from build123d import *

# Parameters (mm, degrees)
ESQUISSE1_W                    = 90
ESQUISSE1_H                    = 60
BOSS_EXTRU_1_DEPTH             = 2.7
ESQUISSE2_W                    = 9
ESQUISSE2_H                    = 2.7
BOSS_EXTRU_2_DEPTH             = 2.7
R_P_TITION_LIN_AIRE1_COUNT     = 3
R_P_TITION_LIN_AIRE1_PITCH     = 18
R_P_TITION_LIN_AIRE1_COL_COUNT = 3
R_P_TITION_LIN_AIRE1_COL_PITCH = 18
ESQUISSE3_W                    = 2.7
ESQUISSE3_H                    = 9.8
ENL_V_MAT_EXTRU_1_DEPTH        = 2.7
R_P_TITION_LIN_AIRE2_COUNT     = 5
R_P_TITION_LIN_AIRE2_PITCH     = 20
SYM_TRIE1_COPY_1_SKETCH_W      = 2.7
SYM_TRIE1_COPY_1_SKETCH_H      = 9.8
SYM_TRIE1_COPY_1_DEPTH         = 2.7
SYM_TRIE1_COPY_2_SKETCH_W      = 2.7
SYM_TRIE1_COPY_2_SKETCH_H      = 9.8
SYM_TRIE1_COPY_2_DEPTH         = 2.7
SYM_TRIE1_COPY_3_SKETCH_W      = 2.7
SYM_TRIE1_COPY_3_SKETCH_H      = 9.8
SYM_TRIE1_COPY_3_DEPTH         = 2.7
SYM_TRIE1_COPY_4_SKETCH_W      = 2.7
SYM_TRIE1_COPY_4_SKETCH_H      = 9.8
SYM_TRIE1_COPY_4_DEPTH         = 2.7
ESQUISSE14_W                   = 30
ESQUISSE14_H                   = 20
ENL_V_MAT_EXTRU_4_DEPTH        = 1


with BuildPart() as part:
    # Esquisse1 → Boss.-Extru.1 (new body)
    with BuildSketch(Plane.XY):
        with Locations((0, -30)):
            Rectangle(ESQUISSE1_W, ESQUISSE1_H)
    extrude(amount=BOSS_EXTRU_1_DEPTH)

    # Esquisse2 → Boss.-Extru.2 (add)
    with BuildSketch(Plane.XY):
        with Locations((0, -61.35)):
            Rectangle(ESQUISSE2_W, ESQUISSE2_H)
    boss_extru_2 = extrude(amount=BOSS_EXTRU_2_DEPTH)

    # Répétition linéaire1: Boss.-Extru.2 ×3
    with Locations(*[(i * R_P_TITION_LIN_AIRE1_PITCH, 0, 0) for i in range(1, R_P_TITION_LIN_AIRE1_COUNT)]):
        add(boss_extru_2)

    # Répétition linéaire1 col: Boss.-Extru.2 ×3
    with Locations(*[(-i * R_P_TITION_LIN_AIRE1_COL_PITCH, 0, 0) for i in range(1, R_P_TITION_LIN_AIRE1_COL_COUNT)]):
        add(boss_extru_2)

    # Esquisse3 → Enlèv. mat.-Extru.1 (cut)
    with BuildSketch(Plane.XY):
        with Locations((43.65, -50)):
            Rectangle(ESQUISSE3_W, ESQUISSE3_H)
    enl_v_mat_extru_1 = extrude(amount=ENL_V_MAT_EXTRU_1_DEPTH, mode=Mode.SUBTRACT)

    # Répétition linéaire2: Enlèv. mat.-Extru.1 ×5
    with Locations(*[(0, i * R_P_TITION_LIN_AIRE2_PITCH, 0) for i in range(1, R_P_TITION_LIN_AIRE2_COUNT)]):
        add(enl_v_mat_extru_1, mode=Mode.SUBTRACT)

    # Symétrie1: Enlèv. mat.-Extru.1 across plane
    add(enl_v_mat_extru_1.mirror(Plane(origin=(0, 0, 0), x_dir=(0, 0, 1), z_dir=(1, 0, 0))), mode=Mode.SUBTRACT)

    # Symétrie1 copy 1 sketch → Symétrie1 copy 1 (cut)
    with BuildSketch(Plane(origin=(0, 20, 0), x_dir=(-1, 0, 0), z_dir=(0, 0, 1))):
        with Locations((43.65, 50)):
            Rectangle(SYM_TRIE1_COPY_1_SKETCH_W, SYM_TRIE1_COPY_1_SKETCH_H)
    extrude(amount=SYM_TRIE1_COPY_1_DEPTH, mode=Mode.SUBTRACT)

    # Symétrie1 copy 2 sketch → Symétrie1 copy 2 (cut)
    with BuildSketch(Plane(origin=(0, 40, 0), x_dir=(-1, 0, 0), z_dir=(0, 0, 1))):
        with Locations((43.65, 50)):
            Rectangle(SYM_TRIE1_COPY_2_SKETCH_W, SYM_TRIE1_COPY_2_SKETCH_H)
    extrude(amount=SYM_TRIE1_COPY_2_DEPTH, mode=Mode.SUBTRACT)

    # Symétrie1 copy 3 sketch → Symétrie1 copy 3 (cut)
    with BuildSketch(Plane(origin=(0, 60, 0), x_dir=(-1, 0, 0), z_dir=(0, 0, 1))):
        with Locations((43.65, 50)):
            Rectangle(SYM_TRIE1_COPY_3_SKETCH_W, SYM_TRIE1_COPY_3_SKETCH_H)
    extrude(amount=SYM_TRIE1_COPY_3_DEPTH, mode=Mode.SUBTRACT)

    # Symétrie1 copy 4 sketch → Symétrie1 copy 4 (cut)
    with BuildSketch(Plane(origin=(0, 80, 0), x_dir=(-1, 0, 0), z_dir=(0, 0, 1))):
        with Locations((43.65, 50)):
            Rectangle(SYM_TRIE1_COPY_4_SKETCH_W, SYM_TRIE1_COPY_4_SKETCH_H)
    extrude(amount=SYM_TRIE1_COPY_4_DEPTH, mode=Mode.SUBTRACT)

    # Esquisse14 → Enlèv. mat.-Extru.4 (cut)
    with BuildSketch(Plane.XY.offset(2.7)):
        with Locations((0, -15)):
            Rectangle(ESQUISSE14_W, ESQUISSE14_H)
    extrude(amount=-ENL_V_MAT_EXTRU_4_DEPTH, mode=Mode.SUBTRACT)


solid = part.part
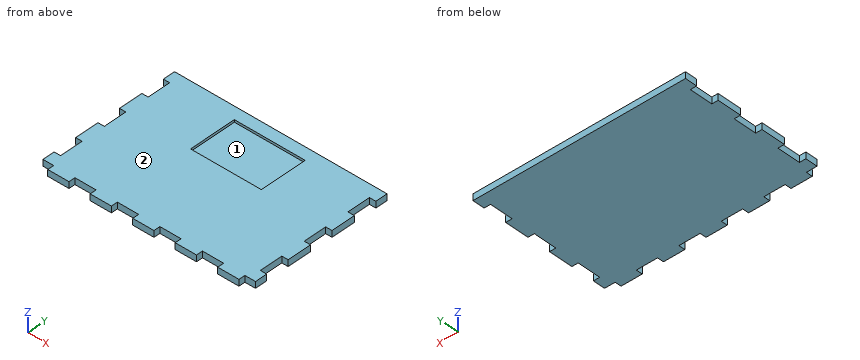
The model under review builds one solid part; all positions refer to its coordinate system, in mm. Face numbers are marked on the shaded views. Give positions to 0.01 mm unless a question says otherwise; leave off trailing zeros. Write each loop counter-clockwise with the first axis right and the second up, starting at its lowest first coordinate (ties: lowest second). Pieces come first, ordered by that corner, then holes.
1. For P1, Ø0.8, axis at y = -29, z = 1.5, coming from the -X side; P2, Ø1, axis at x = -6, z = 1, coming from the -Y side; P3, Ø1.4, axis at y = -50, z = 1, coming from the +X side, all flat-tipped, find the tip position at first contact; note any pin that passes through.
2. Add section B-B, the plane y = -18. Write out the cut boundary in (x, z).
3. Add section C-C, the plane y = -31. Write out the cut boundary in (x, z), plus the area to 3 significant figures.
4. Wall thickness on L1, parallel to X at y = -28.5, z = 1.35; L2, parallel to Y at x = 27.5, z = 1.85; L3, parallel to Z at x = -6, y = -7: over which ranges is each line inside the solid? List them lowest first.
5. Add section A-A, the plane x = -2. Write out the cut boundary in (y, z), plus the area to 3 significant figures.
6. Draft analysis for pull direction Y (two halves, no side actions). For the marked faces 1 and 2, state which applies: +Y half, -Y half, draft (parallel to the pull), parting line (faces both ways), or undercut.
Worked answers:
1. P1: stops at x = -42.3
1. P2: stops at y = -60
1. P3: stops at x = 42.3
2. outline: (-45, 0) - (45, 0) - (45, 2.7) - (15, 2.7) - (15, 1.7) - (-15, 1.7) - (-15, 2.7) - (-45, 2.7) - close
3. outline: (-42.3, 0) - (42.3, 0) - (42.3, 2.7) - (-42.3, 2.7) - close
3. area: 228 mm2
4. L1: x = -42.3 to 42.3
4. L2: y = -60 to 0
4. L3: z = 0 to 1.7
5. outline: (-62.7, 0) - (0, 0) - (0, 2.7) - (-5, 2.7) - (-5, 1.7) - (-25, 1.7) - (-25, 2.7) - (-62.7, 2.7) - close
5. area: 149 mm2
6. face 1: undercut
6. face 2: draft
